Solid Edge part; units mm, degrees
sketch "Sketch1" plane through (0, 0, 0) normal (0, 0, 1) x (1, 0, 0)
  line L0 (0, 0) -> (60, 0)
  line L1 (60, 0) -> (60, 30)
  line L2 (60, 30) -> (0, 30)
  line L3 (0, 30) -> (0, 0)
extrude "Protrusion1" add sketch "Sketch1" along normal blind 2
sketch "Sketch2" plane through (20, 0, 0) normal (1, 0, 0) x (0, 1, 0)
  circle A0 centre (0, 1) radius 5
extrude "拉伸_2" add sketch "Sketch2" along normal blind 20
sketch "Sketch3" plane through (20, 0, 0) normal (1, 0, 0) x (0, 1, 0)
  circle A0 centre (0, 1) radius 3.2
extrude "拉伸除料_1" cut sketch "Sketch3" along normal blind 20
Verification items for the finished model (mm, model axes). A direction names the side the tool comes from. Give positions to 0.01 mm unless a question says otherwise; leave off trailing zeros. Loops run counter-clockwise (first coordinate to the right, second up) from the corner with the lowest first, then second, coordinate; pieces in that order, holes last.
1. Release check for a two-part mould opening along Z. For faces 3 (the flat face through (60, 15, 1)), 4 (the cylindrical face through (29.86, -0.694, 4.124)), 5 (the cylindrical face through (30, -5, 1)) record: +Z half, -Z half, draft (parallel to the pull), parting line (faces both ways), or undercut.
Derived:
face 3: draft
face 4: undercut
face 5: parting line
2. Cross-section at A-A on z = 1. Record the cut outline in (x, y).
Derived:
outline: (0, 0) - (20, 0) - (20, 3.2) - (40, 3.2) - (40, 0) - (60, 0) - (60, 30) - (0, 30) - close; (20, -5) - (40, -5) - (40, -3.2) - (20, -3.2) - close
3. Cross-section at C-C on y = 20.5. Record the cut outline in (x, z), and give its area (3 significant figures).
Derived:
outline: (0, 0) - (60, 0) - (60, 2) - (0, 2) - close
area: 120 mm2
4. Cross-section at B-B on z = 5. Record the cut outline in (x, y), and give its area (3 significant figures).
Derived:
outline: (20, -3) - (40, -3) - (40, 3) - (20, 3) - close
area: 120 mm2
5. Tool access check on faces 1 (the flat face through (40, 2, 1)), 2 (the flat face through (10, 0, 1)). Record the directions out of +Z, -Z, +X, -X, +Y, -Y that give a thin tool (end or side, any length) a straight path to the whole face; none if there is none.
Derived:
face 1: none
face 2: +Z, -Z, +X, -X, -Y
6. Go/stop test with flat-tipped pins: P1, Ø12, axis at x = 39, y = 6.5, coming from the -Z side; P2, Ø1, axis at x = 25, y = 22.5, coming from the -Z side; P3, Ø0.6, axis at x = 11, z = 1.5, coming from the -Y side. Record where each tip stops, or that it passes through.
Derived:
P1: stops at z = -3.97
P2: stops at z = 0
P3: stops at y = 0
7. Material ranges on probe 1 along Y at (x, z) = (31.75, 1); probe 2 along Z at (x, y) = (34.5, 0); probe 3 along X at (y, z) = (1, 0.5), recorded low to high.
Derived:
probe 1: y = -5 to -3.2, 3.2 to 30
probe 2: z = -4 to -2.2, 4.2 to 6
probe 3: x = 0 to 20, 40 to 60
